```python
from build123d import *

# Parameters (mm, degrees)
EXTRUDE1_DEPTH       = 39.5
SKETCH2_W            = 19.5
SKETCH2_H            = 8.1
EXTRUDE2_DEPTH       = 40.5
EXTRUDE3_START       = 1.5
SKETCH3_R            = 7.5
EXTRUDE3_DEPTH       = 1.5
HOLEWZD1_D           = 10
HOLEWZD1_DEPTH       = 1.5
SKETCH6_W            = 4.5
SKETCH6_H            = 1.5
HOLEWZD2_D           = 8
HOLEWZD2_DEPTH       = 81.500025
HOLEWZD3_D           = 6.5
HOLEWZD3_CBORE_D     = 11
HOLEWZD3_CBORE_DEPTH = 4.4
FILLET1_R            = 1
FILLET2_R            = 3


with BuildPart() as part:
    # Sketch1 → Extrude1 (new body)
    with BuildSketch(Plane(origin=(0, 40, 0), x_dir=(1, 0, 0), z_dir=(0, 1, 0))):
        with BuildLine():
            Line((27.5, 8.1), (2, 8.1))
            Line((2, 8.1), (2, 7.228416147))
            ThreePointArc((2, 7.228416147), (-5.968668193, -4.541475531), (7.5, 0))
            Line((7.5, 0), (27.5, 0))
            Line((27.5, 0), (27.5, 8.1))
        make_face()
    extrude(amount=-EXTRUDE1_DEPTH)

    # Sketch2 → Extrude2 (add)
    with BuildSketch(Plane.XZ.offset(-0.5)):
        with Locations((17.75, -4.05)):
            Rectangle(SKETCH2_W, SKETCH2_H)
    extrude(amount=EXTRUDE2_DEPTH)

    # Sketch3 → Extrude3 (add)
    with BuildSketch(Plane(origin=(0, 40, 0), x_dir=(-1, 0, 0), z_dir=(0, 1, 0)).offset(EXTRUDE3_START)):
        with Locations(Location((0, 0, 0), (0, 0, 90))):
            Circle(SKETCH3_R)
    extrude(amount=-EXTRUDE3_DEPTH)

    # HoleWzd1
    with Locations(Plane(origin=(0, 41.5, 0), x_dir=(1, 0, 0), z_dir=(0, 1, 0))):
        with Locations((0, 0)):
            Hole(HOLEWZD1_D / 2, depth=HOLEWZD1_DEPTH)

    # Sketch6 → Revolve1 (revolve)
    with BuildSketch(Plane(origin=(0, 0, 0), x_dir=(-1, 0, 0), z_dir=(0, 0, -1)), mode=Mode.PRIVATE) as revolve1_sk:
        with Locations((-2.25, 40.75)):
            Rectangle(SKETCH6_W, SKETCH6_H)
    revolve(revolve1_sk.sketch.rotate(Axis((0, 40, 0), (0, 1, 0)), 270), axis=Axis((0, 40, 0), (0, 1, 0)))

    # HoleWzd2
    with Locations(Plane(origin=(0, 41.5, 0), x_dir=(1, 0, 0), z_dir=(0, 1, 0))):
        with Locations((0, 0)):
            Hole(HOLEWZD2_D / 2, depth=HOLEWZD2_DEPTH)

    # HoleWzd3 (through all)
    with Locations(Plane.XY):
        with Locations((15.5, 21.5), (15.5, -21.5)):
            CounterBoreHole(HOLEWZD3_D / 2, HOLEWZD3_CBORE_D / 2, HOLEWZD3_CBORE_DEPTH)

    # Fillet1
    fillet1_edges = [part.edges().sort_by_distance(p)[0] for p in [
        (27.5, 0, 0),
    ]]
    fillet(fillet1_edges, radius=FILLET1_R)

    # Fillet2
    # the kernel refuses this fillet: 3 mm, written as the material it takes off along each edge
    with BuildSketch(Plane(origin=(27.5, 40, 6.5), x_dir=(-1, 0, 0), z_dir=(0, 0, -1))) as fillet2_piece_1:
        with BuildLine():
            CenterArc((FILLET2_R, -FILLET2_R), FILLET2_R, 90, 90)
            Line((0, -FILLET2_R), (0, 0))
            Line((0, 0), (FILLET2_R, 0))
        make_face()
    extrude(amount=22.1, mode=Mode.SUBTRACT)
    with BuildSketch(Plane(origin=(27.5, -40, 6.5), x_dir=(-1, 0, 0), z_dir=(0, 0, -1))) as fillet2_piece_2:
        with BuildLine():
            CenterArc((FILLET2_R, FILLET2_R), FILLET2_R, 180, 90)
            Line((0, FILLET2_R), (0, 0))
            Line((0, 0), (FILLET2_R, 0))
        make_face()
    extrude(amount=22.1, mode=Mode.SUBTRACT)


solid = part.part
```
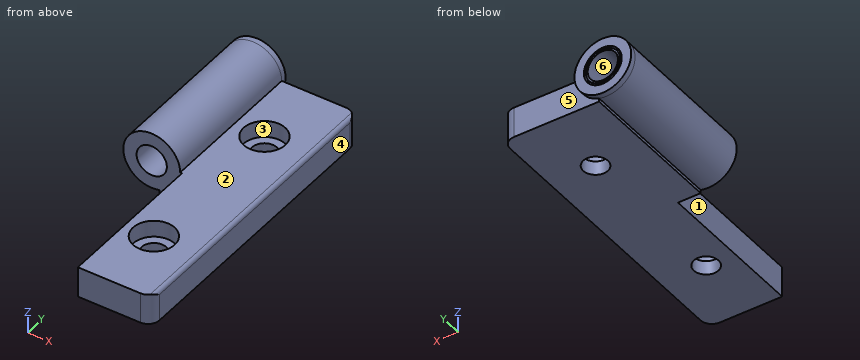
Work out the finished part from the listing and answer in its coordinate system (mm). Face numbers are marked on the shaded views. A direction names the side the tool comes from. Give positions to 0.01 mm unless a question says otherwise; leave off trailing zeros. Order: outer loops, then holes, each group sorted by start corner. A loop starts at its lowest first (then second) coordinate and runs counter-clockwise, first axis right, second up. Notation, with made-up numbers: (-22.5, 59) -> (28.5, 59) arc R21 cw to (28.5, 68) -> close; hole circle Ø7 at (5.25, -33). An arc over 180 degrees is marked (long way). Answer as CSV lines item,"result". Start each with the question number.
(1) Section A-A, the plane y = 21.5 is taken. Write down the section's boundary in (x, z).
(2) Section B-B, the plane x = 15.5 is taken. Write down the section's boundary in (y, z), plus the area to 3 significant figures.
(3) Section D-D, the plane y = -21.5 is taken. Write down the section's boundary in (x, z).
(4) Each of these flat-tipped pins is pushed along its axis until it touches: pin 1 Ø10 at (x, y) = (2.5, -18.5) entering from +Z; pin 2 Ø9 at (y, z) = (-27.5, -5) entering from -X; pin 3 Ø5.5 at (x, y) = (18.5, -15) entering from +Z; pin 4 Ø1 at (y, z) = (18, -3) entering from -X. Where does it stop, or does it pass through?
(5) Section C-C, the plane x = 0 is taken. Write down the section's boundary in (y, z), plus the area to 4 significant figures.
(6) Consider line 1 along Y through (x, z) = (15.5, -1.9); line 2 along Y through (x, z) = (14.5, -6.25); line 3 along Z through (x, y) = (25, 9.5). Determine where each line is inside the solid, lowest interval first.
(7) For a pull along X with two mould halves and no side action, classify the marked faces 4, 5 and 6 as released by +X, released by -X, zero draft, split by the parting line, or undercut.
(8) Which of the six approach directions +Z, -Z, +X, -X, +Y, -Y give full straight-line access (tool end or side, diameter ignored) to the marked faces 1, 2 and 3?
Entries:
1,outline,"(2, -8.1) -> (12.25, -8.1) -> (12.25, -4.4) -> (10, -4.4) -> (10, 0) -> (7.5, 0) arc R7.5 ccw (long way) to (2, -7.23) -> close; (18.75, -8.1) -> (27.5, -8.1) -> (27.5, -1) arc R1 ccw to (26.5, 0) -> (21, 0) -> (21, -4.4) -> (18.75, -4.4) -> close; hole circle Ø8 at (0, 0)"
2,outline,"(-40, -8.1) -> (-24.75, -8.1) -> (-24.75, -4.4) -> (-27, -4.4) -> (-27, 0) -> (-40, 0) -> close; (-18.25, -8.1) -> (18.25, -8.1) -> (18.25, -4.4) -> (16, -4.4) -> (16, 0) -> (-16, 0) -> (-16, -4.4) -> (-18.25, -4.4) -> close; (24.75, -8.1) -> (40, -8.1) -> (40, 0) -> (27, 0) -> (27, -4.4) -> (24.75, -4.4) -> close"
2,area,"503 mm²"
3,outline,"(8, -8.1) -> (12.25, -8.1) -> (12.25, -4.4) -> (10, -4.4) -> (10, 0) -> (8, 0) -> close; (18.75, -8.1) -> (27.5, -8.1) -> (27.5, -1) arc R1 ccw to (26.5, 0) -> (21, 0) -> (21, -4.4) -> (18.75, -4.4) -> close"
4,pin 1,"through"
4,pin 2,"x = 8"
4,pin 3,"z = 0"
4,pin 4,"x = -7.07"
5,outline,"(0.5, -7.5) -> (41.5, -7.5) -> (41.5, -5) -> (40, -5) -> (40, -4.5) -> (41.5, -4.5) -> (41.5, -4) -> (0.5, -4) -> close; (0.5, 4) -> (41.5, 4) -> (41.5, 4.5) -> (40, 4.5) -> (40, 5) -> (41.5, 5) -> (41.5, 7.5) -> (0.5, 7.5) -> close"
5,area,"285.5 mm²"
6,line 1,"-40 to -27, -16 to 16, 27 to 40"
6,line 2,"-40 to -24.59, -18.41 to 18.41, 24.59 to 40"
6,line 3,"-8.1 to 0"
7,face 4,"released by +X"
7,face 5,"zero draft"
7,face 6,"undercut"
8,face 1,"+Z, -Z, -X, -Y"
8,face 2,"+Z, +X, +Y, -Y"
8,face 3,"+Z"
